The listing builds one solid part. Answer for the finished solid, in the listing's coordinates (mm). A direction names the side the tool comes from. Coordinates: 2 decimals unless noted, no trailing zeros. Answer in a Markdown table with one row per item.
```python
from build123d import *

# Parameters (mm, degrees)
SKETCH_1_R          = 1
EXTRUDE_1_DEPTH     = 2
SKETCH_2_R          = 1
CUT_EXTRUDE_1_DEPTH = 10


with BuildPart() as part:
    # 草圖1 → 填料-伸長1 (new body)
    with BuildSketch(Plane.XY):
        with BuildLine():
            Line((23.861531606, 13.243524775), (25.861531606, 13.243524775))
            ThreePointArc((25.861531606, 13.243524775), (26.568638387, 13.536417994), (26.861531606, 14.243524775))
            Line((26.861531606, 14.243524775), (26.861531606, 16.243524775))
            Line((26.861531606, 16.243524775), (80.861531606, 16.243524775))
            Line((80.861531606, 16.243524775), (81.861531606, 16.243524775))
            Line((81.861531606, 16.243524775), (81.861531606, 15.243524775))
            Line((81.861531606, 15.243524775), (81.861531606, -7.006475225))
            Line((81.861531606, -7.006475225), (79.861531606, -7.006475225))
            ThreePointArc((79.861531606, -7.006475225), (79.154424825, -7.299368444), (78.861531606, -8.006475225))
            Line((78.861531606, -8.006475225), (78.861531606, -10.006475225))
            ThreePointArc((78.861531606, -10.006475225), (79.154424825, -10.713582006), (79.861531606, -11.006475225))
            Line((79.861531606, -11.006475225), (81.861531606, -11.006475225))
            Line((81.861531606, -11.006475225), (81.861531606, -39.006475225))
            Line((81.861531606, -39.006475225), (81.861531606, -40.006475225))
            Line((81.861531606, -40.006475225), (80.861531606, -40.006475225))
            Line((80.861531606, -40.006475225), (61.861531606, -40.006475225))
            Line((61.861531606, -40.006475225), (61.861531606, -38.006475225))
            ThreePointArc((61.861531606, -38.006475225), (61.568638387, -37.299368444), (60.861531606, -37.006475225))
            Line((60.861531606, -37.006475225), (58.861531606, -37.006475225))
            ThreePointArc((58.861531606, -37.006475225), (58.154424825, -37.299368444), (57.861531606, -38.006475225))
            Line((57.861531606, -38.006475225), (57.861531606, -40.006475225))
            Line((57.861531606, -40.006475225), (-8.138468394, -40.006475225))
            Line((-8.138468394, -40.006475225), (-8.138468394, -38.006475225))
            ThreePointArc((-8.138468394, -38.006475225), (-8.431361613, -37.299368444), (-9.138468394, -37.006475225))
            Line((-9.138468394, -37.006475225), (-11.138468394, -37.006475225))
            ThreePointArc((-11.138468394, -37.006475225), (-11.845575175, -37.299368444), (-12.138468394, -38.006475225))
            Line((-12.138468394, -38.006475225), (-12.138468394, -40.006475225))
            Line((-12.138468394, -40.006475225), (-31.138468394, -40.006475225))
            Line((-31.138468394, -40.006475225), (-32.138468394, -40.006475225))
            Line((-32.138468394, -40.006475225), (-32.138468394, -39.006475225))
            Line((-32.138468394, -39.006475225), (-32.138468394, -11.006475225))
            Line((-32.138468394, -11.006475225), (-30.138468394, -11.006475225))
            ThreePointArc((-30.138468394, -11.006475225), (-29.431361613, -10.713582006), (-29.138468394, -10.006475225))
            Line((-29.138468394, -10.006475225), (-29.138468394, -8.006475225))
            ThreePointArc((-29.138468394, -8.006475225), (-29.431361613, -7.299368444), (-30.138468394, -7.006475225))
            Line((-30.138468394, -7.006475225), (-32.138468394, -7.006475225))
            Line((-32.138468394, -7.006475225), (-32.138468394, 15.243524775))
            Line((-32.138468394, 15.243524775), (-32.138468394, 16.243524775))
            Line((-32.138468394, 16.243524775), (-31.138468394, 16.243524775))
            Line((-31.138468394, 16.243524775), (22.861531606, 16.243524775))
            Line((22.861531606, 16.243524775), (22.861531606, 14.243524775))
            ThreePointArc((22.861531606, 14.243524775), (23.154424825, 13.536417994), (23.861531606, 13.243524775))
        make_face()
        with Locations((55.861531606, -36.006475225)):
            Circle(SKETCH_1_R, mode=Mode.SUBTRACT)
        with Locations((77.861531606, -5.006475225)):
            Circle(SKETCH_1_R, mode=Mode.SUBTRACT)
        with Locations((-6.138468394, -36.006475225)):
            Circle(SKETCH_1_R, mode=Mode.SUBTRACT)
        with Locations((28.861531606, 12.243524775)):
            Circle(SKETCH_1_R, mode=Mode.SUBTRACT)
        with Locations((20.861531606, 12.243524775)):
            Circle(SKETCH_1_R, mode=Mode.SUBTRACT)
        with Locations((-28.138468394, -5.006475225)):
            Circle(SKETCH_1_R, mode=Mode.SUBTRACT)
        with Locations((-28.138468394, -13.006475225)):
            Circle(SKETCH_1_R, mode=Mode.SUBTRACT)
        with Locations((77.861531606, -13.006475225)):
            Circle(SKETCH_1_R, mode=Mode.SUBTRACT)
        with Locations((-14.138468394, -36.006475225)):
            Circle(SKETCH_1_R, mode=Mode.SUBTRACT)
        with Locations((63.861531606, -36.006475225)):
            Circle(SKETCH_1_R, mode=Mode.SUBTRACT)
    extrude(amount=EXTRUDE_1_DEPTH)

    # 草圖2 → 除料-伸長1 (cut)
    with BuildSketch(Plane.XY.offset(2)):
        with Locations((7.861531606, -21.006475225)):
            Circle(SKETCH_2_R)
        with Locations((41.861531606, -21.006475225)):
            Circle(SKETCH_2_R)
    extrude(amount=-CUT_EXTRUDE_1_DEPTH, mode=Mode.SUBTRACT)


solid = part.part
```
(1) Find the intervals of material crossed by line 1 along X through (y, z) = (-36, 0.7); line 2 along Y through (x, z) = (-6, 1.2); line 3 along Y through (x, z) = (63, 0.9), in increasing order. Write a range as from..to.
Check values:
| item | result |
|---|---|
| line 1 | -32.14..-15.14, -13.14..-7.14, -5.14..54.86, 56.86..62.86, 64.86..81.86 |
| line 2 | -40.01..-37, -35.02..16.24 |
| line 3 | -40.01..-36.51, -35.5..16.24 |
(2) For a pull along Y with two mould halves and no side action, classify faces 1 (the flat face through (25, -40.006, 1)), 2 (the cylindrical face through (6.862, -20.963, 1.014)), 3 (the flat face through (22.862, 15, 1)) as released by +Y, released by -Y, zero draft, split by the parting line, or undercut.
Check values:
| item | result |
|---|---|
| face 1 | released by -Y |
| face 2 | undercut |
| face 3 | zero draft |
(3) Which of the six approach directions +Z, -Z, +X, -X, +Y, -Y give full straight-line access (tool end or side, diameter ignored) to faces 4 (the flat face through (61.862, -39, 1)), 5 (the flat face through (-31, -7.006, 1)), 6 (the flat face through (81, -11.006, 1))?
Check values:
| item | result |
|---|---|
| face 4 | +Z, -Z, -Y |
| face 5 | +Z, -Z, -X |
| face 6 | +Z, -Z, +X |
(4) Flat-ended cylindrical pins translate along their axes: pin 1 (2.5 mm diameter, centred on x = -14.14, y = -36.01, fed in from +Z); pin 2 (1.8 mm diameter, centred on x = 77.86, y = -13.01, fed in from +Z). Find the tip coordinate at first contact, or state that the pin passes through.
Check values:
| item | result |
|---|---|
| pin 1 | z = 2 |
| pin 2 | through |
